from build123d import *

# Parameters (mm, degrees)
F0_W     = 50.8
F0_H     = 50.8
F0_R     = 9.525
F1_DEPTH = 50.8
F2_R     = 9.525
F3_DEPTH = 50.8
F4_R     = 9.525
F5_DEPTH = 50.8


with BuildPart() as f1:
    # F0 (on Front) → F1 (new body)
    with BuildSketch(Plane.XZ):
        with Locations((0, -4.425067)):
            Rectangle(F0_W, F0_H)
        with Locations((0, -4.425067)):
            Circle(F0_R, mode=Mode.SUBTRACT)
    extrude(amount=F1_DEPTH)

    # F2 (on face) → F3 (cut)
    with BuildSketch(Plane(origin=(0, 0, -29.825067), x_dir=(1, 0, 0), z_dir=(0, 0, -1))):
        with Locations((0, 25.4)):
            Circle(F2_R)
    extrude(amount=-F3_DEPTH, mode=Mode.SUBTRACT)

    # F4 (on face) → F5 (cut)
    with BuildSketch(Plane.YZ.offset(25.4)):
        with Locations((-25.4, -4.425067)):
            Circle(F4_R)
    extrude(amount=-F5_DEPTH, mode=Mode.SUBTRACT)


solid = f1.part
Geometry: final body of the model. Coordinates: model frame, mm. Round coordinates to 2 decimals unless told otherwise and drop trailing zeros. Order: outer loops, then holes, each group sorted by start corner. A loop starts at its lowest first (then second) coordinate and runs counter-clockwise, first axis right, second up. Notation, with made-up numbers: (12.5, 16.5) -> (31.5, 16.5) arc R21 cw to (31.5, 35.5) -> close; hole circle Ø7 at (17.5, 59.25). An arc over 180 degrees is marked (long way). Put each result on its own line as item: value. Start each with the question number.
Q1. First-contact query: pin 1 (4 mm diameter, centred on x = 1.5, y = -17.5, fed in from -Z). Flat tip, straight axial feed; report the tip coordinate or a pass-through.
Q2. Section B-B on y = -25.4. Return the cut outline in (x, z) (3 decimals).
Q3. Section C-C on z = -19. Return the cut outline in (x, y) (3 decimals), and give its area (3 significant figures).
Q4. Section A-A on x = 0. Return the cut outline in (y, z) (3 decimals), and give its area (3 significant figures).
Q5. Pull-direction query (X, two-part tool) for faces 1 (the cylindrical face through (-9.516, -9.202, -4.006)), 2 (the cylindrical face through (-15.937, -34.916, -4.006)), 3 (the cylindrical face through (-9.516, -25.819, 11.512)), 4 (the flat face through (25.4, -25, -16)); classes: +X half, -X half, draft (parallel to the pull), parting line (faces both ways), or undercut.
Q6. Section D-D on x = -15.5. Return the cut outline in (y, z) (3 decimals).
Q7. Line query: probe 1 along Z at (x, y) = (-14, -25); probe 2 along X at (y, z) = (-25.4, -15) (3 decimals); probe 3 along Y at (x, z) = (0, -25) (3 decimals). Output: solid intervals per line, ascending.
Ans:
1. pin 1: stops at z = -29.83
2. outline: (-25.4, -29.825) -> (-9.525, -29.825) -> (-9.525, -13.95) -> (-25.4, -13.95) -> close; (-25.4, 5.1) -> (-9.525, 5.1) -> (-9.525, 20.975) -> (-25.4, 20.975) -> close; (9.525, -29.825) -> (25.4, -29.825) -> (25.4, -13.95) -> (9.525, -13.95) -> close; (9.525, 5.1) -> (25.4, 5.1) -> (25.4, 20.975) -> (9.525, 20.975) -> close
3. outline: (-25.4, -50.8) -> (25.4, -50.8) -> (25.4, 0) -> (-25.4, 0) -> close; hole circle Ø19.05 at (0, -25.4)
3. area: 2,300 mm2
4. outline: (-50.8, -29.825) -> (-34.925, -29.825) -> (-34.925, -13.95) -> (-50.8, -13.95) -> close; (-50.8, 5.1) -> (-34.925, 5.1) -> (-34.925, 20.975) -> (-50.8, 20.975) -> close; (-15.875, -29.825) -> (0, -29.825) -> (0, -13.95) -> (-15.875, -13.95) -> close; (-15.875, 5.1) -> (0, 5.1) -> (0, 20.975) -> (-15.875, 20.975) -> close
4. area: 1,010 mm2
5. face 1: undercut
5. face 2: draft
5. face 3: undercut
5. face 4: +X half
6. outline: (-50.8, -29.825) -> (0, -29.825) -> (0, 20.975) -> (-50.8, 20.975) -> close; hole circle Ø19.05 at (-25.4, -4.425)
7. probe 1: z = -29.83 to -13.94, 5.09 to 20.97
7. probe 2: x = -25.4 to -9.525, 9.525 to 25.4
7. probe 3: y = -50.8 to -34.925, -15.875 to 0
